Here's how the part is built. I have some questions about the finished solid (model axes, mm). A direction names the side the tool comes from. Round coordinates to 2 decimals unless told otherwise and drop trailing zeros. Write each loop counter-clockwise with the first axis right and the second up, starting at its lowest first coordinate (ties: lowest second). Pieces come first, ordered by that corner, then holes. Notation, with made-up numbers: (81, 19.5) - (105, 19.5) arc R33 cw to (105, 47.5) - close; hole circle Ø1 at (-10, -3.75). An arc over 180 degrees is marked (long way). One line per item, written item: value. Start each with the question number.
Item 1: Imagine slicing it at D-D, the plane y = -0.95. Count the separate pieces of the cut face and the enclosed holes in it, then the cut area to 3 significant figures.
Item 2: For P1, Ø1, axis at y = -1.5, z = 40, coming from the -X side; P2, Ø3, axis at x = 23.82, z = 13.75, coming from the -Y side; P3, Ø0.6, axis at x = 46, y = -1.5, coming from the +Z side; P4, Ø1, axis at x = -43.5, y = -1, coming from the -Z side, each with a flat end and sliding along its axis, tell me the tip position at first contact or that it passes through.
Item 3: If I drill on line 1 (X direction, y = -1.2, z = 13.75); line 2 (X direction, y = -0.85, z = 36); line 3 (Z direction, x = -32.5, y = -0.9), over which ranges is the centre line in solid material (lowest first)?
Item 4: Thinking about a two-plate mould opening in X: for faces 5 (the face through (32.098, -1.014, -41.229)), 6 (the face through (-8.19, -0.99, 29.12)), 7 (the face through (-29, -1, 29)), which applies, released by +X, released by -X, zero draft, split by the parting line, or undercut?
Item 5: For faces 1 (the face through (29, -1, 29)), 2 (the face through (-14.8, -0.99, -26.38)), 3 (the face through (-29, -1, -29)), 4 (the face through (29.12, -0.99, 8.19)), which set-ups out of +Z, -Z, +X, -X, +Y, -Y let a thin tool reach every point of the face, with its end or its side?
Item 6: Imagine slicing it at C-C, the plane x = -42. Please give me the cut outline in (y, z).
Item 7: Imagine slicing it at A-A, the plane x = -11. Please give me the cut outline in (y, z).
Item 8: Imagine slicing it at B-B, the plane x = -24. Please give me the cut outline in (y, z), then the cut area to 3 significant figures.
```python
from build123d import *

# Parameters (mm, degrees)
SKETCH1_R           = 30.25
SKETCH1_R_2         = 25.25
EXTRUDE_THIN1_DEPTH = 2
SKETCH2_R           = 1.65
CUT_EXTRUDE3_DEPTH  = 10
BOSS_EXTRUDE1_DEPTH = 2


with BuildPart() as part:
    # Sketch1 → Extrude-Thin1 (new body)
    with BuildSketch(Plane(origin=(0, 0, 0), x_dir=(1, 0, 0), z_dir=(0, 1, 0))):
        Circle(SKETCH1_R)
        Circle(SKETCH1_R_2, mode=Mode.SUBTRACT)
    extrude(amount=-EXTRUDE_THIN1_DEPTH)

    # Sketch2 → Cut-Extrude3 (cut)
    with BuildSketch(Plane(origin=(0, 0, 0), x_dir=(1, 0, 0), z_dir=(0, 1, 0))):
        with Locations((0, 27.5)):
            Circle(SKETCH2_R)
        with Locations((23.815698604, -13.75)):
            Circle(SKETCH2_R)
        with Locations((-23.815698604, -13.75)):
            Circle(SKETCH2_R)
    extrude(amount=-CUT_EXTRUDE3_DEPTH, mode=Mode.SUBTRACT)

    # Sketch5 → Boss-Extrude1 (add)
    with BuildSketch(Plane.XZ.offset(2)):
        with BuildLine():
            Line((0, 52.25), (0, 30.25))
            ThreePointArc((0, 30.25), (3.686547638, 30.024521087), (7.318137342, 29.35144572))
            Line((7.318137342, 29.35144572), (12.640419045, 50.697951698))
            ThreePointArc((12.640419045, 50.697951698), (6.367673193, 51.860536423), (0, 52.25))
        make_face()
        with BuildLine():
            Line((36.946329317, 36.946329317), (21.389980131, 21.389980131))
            ThreePointArc((21.389980131, 21.389980131), (23.837325297, 18.623759629), (25.929310846, 15.579901766))
            Line((25.929310846, 15.579901766), (44.786991462, 26.910739414))
            ThreePointArc((44.786991462, 26.910739414), (41.173561876, 32.168312086), (36.946329317, 36.946329317))
        make_face()
        with BuildLine():
            Line((52.25, 0), (30.25, 0))
            ThreePointArc((30.25, 0), (30.024521087, -3.686547638), (29.35144572, -7.318137342))
            Line((29.35144572, -7.318137342), (50.697951698, -12.640419045))
            ThreePointArc((50.697951698, -12.640419045), (51.860536423, -6.367673193), (52.25, 0))
        make_face()
        with BuildLine():
            Line((36.946329317, -36.946329317), (21.389980131, -21.389980131))
            ThreePointArc((21.389980131, -21.389980131), (18.623759629, -23.837325297), (15.579901766, -25.929310846))
            Line((15.579901766, -25.929310846), (26.910739414, -44.786991462))
            ThreePointArc((26.910739414, -44.786991462), (32.168312086, -41.173561876), (36.946329317, -36.946329317))
        make_face()
        with BuildLine():
            Line((0, -52.25), (0, -30.25))
            ThreePointArc((0, -30.25), (-3.686547638, -30.024521087), (-7.318137342, -29.35144572))
            Line((-7.318137342, -29.35144572), (-12.640419045, -50.697951698))
            ThreePointArc((-12.640419045, -50.697951698), (-6.367673193, -51.860536423), (0, -52.25))
        make_face()
        with BuildLine():
            Line((-36.946329317, -36.946329317), (-21.389980131, -21.389980131))
            ThreePointArc((-21.389980131, -21.389980131), (-23.837325297, -18.623759629), (-25.929310846, -15.579901766))
            Line((-25.929310846, -15.579901766), (-44.786991462, -26.910739414))
            ThreePointArc((-44.786991462, -26.910739414), (-41.173561876, -32.168312086), (-36.946329317, -36.946329317))
        make_face()
        with BuildLine():
            Line((-52.25, 0), (-30.25, 0))
            ThreePointArc((-30.25, 0), (-30.024521087, 3.686547638), (-29.35144572, 7.318137342))
            Line((-29.35144572, 7.318137342), (-50.697951698, 12.640419045))
            ThreePointArc((-50.697951698, 12.640419045), (-51.860536423, 6.367673193), (-52.25, 0))
        make_face()
        with BuildLine():
            Line((-36.946329317, 36.946329317), (-21.389980131, 21.389980131))
            ThreePointArc((-21.389980131, 21.389980131), (-18.623759629, 23.837325297), (-15.579901766, 25.929310846))
            Line((-15.579901766, 25.929310846), (-26.910739414, 44.786991462))
            ThreePointArc((-26.910739414, 44.786991462), (-32.168312086, 41.173561876), (-36.946329317, 36.946329317))
        make_face()
    extrude(amount=-BOSS_EXTRUDE1_DEPTH)


solid = part.part
```
Values follow:
1. separate pieces: 1
1. enclosed holes: 4
1. area: 2,620 mm^2
2. P1: stops at x = -34.2
2. P2: passes through
2. P3: stops at z = 0
2. P4: stops at z = -29.68
3. line 1: x = -26.94 to -25.47, -22.17 to -21.18, 21.18 to 22.17, 25.47 to 26.94
3. line 2: x = -36 to -21.63, 0 to 8.98, 36 to 37.87
3. line 3: z = -32.5 to -19.53, 0 to 8.1, 32.5 to 40.91
4. face 5: released by +X
4. face 6: undercut
4. face 7: released by -X
5. face 1: +Z, +Y, -Y
5. face 2: +Y, -Y
5. face 3: -Z, +Y, -Y
5. face 4: +X, +Y, -Y
6. outline: (-2, -31.08) - (0, -31.08) - (0, -25.24) - (-2, -25.24) - close; (-2, 0) - (0, 0) - (0, 10.47) - (-2, 10.47) - close
7. outline: (-2, -51.08) - (0, -51.08) - (0, -44.12) - (-2, -44.12) - close; (-2, -28.18) - (0, -28.18) - (0, -22.73) - (-2, -22.73) - close; (-2, 22.73) - (0, 22.73) - (0, 28.18) - (-2, 28.18) - close
8. outline: (-2, -24) - (0, -24) - (0, -7.85) - (-2, -7.85) - close; (-2, 7.85) - (0, 7.85) - (0, 12.11) - (-2, 12.11) - close; (-2, 15.39) - (0, 15.39) - (0, 18.41) - (-2, 18.41) - close; (-2, 24) - (0, 24) - (0, 39.94) - (-2, 39.94) - close
8. area: 78.8 mm^2
